Part print with two shaded views. Sizes in mm from the minimum x, y, z corner. Round coordinates to 2 decimals unless told otherwise and drop trailing zeros. Loops run counter-clockwise (first coordinate to the right, second up) from the corner with the lowest first, then second, coordinate; pieces in that order, holes last. Notation, with made-up numbers: M 68.25,13 L 97.25,13 A9 ccw 97.25,26 Z; hole C 56.25,70 d9. An arc over 180 degrees is marked long. Use a Markdown table: item, result. Add a question column.
Item 1: Pin check, flat tips, straight feed: P1, Ø5, axis at x = 185.5, z = 11, coming from the -Y side; P2, Ø10, axis at y = 18.5, z = 2.5, coming from the -X side; P3, Ø5.5, axis at y = 42, z = 2, coming from the +X side. Stop position of each tip, or through.
Item 2: Saw through at C-C on y = 43. Write the cut outline in (x, z), then the cut area to 3 significant figures.
Item 3: Saw through at A-A on x = 175. Write the cut outline in (y, z).
Item 4: Saw through at D-D on x = 67. Write the cut outline in (y, z), then the cut area to 3 significant figures.
Item 5: Wall check: L1, parallel to Y at x = 182.3, z = 3.65; L2, parallel to Z at x = 178.5, y = 80; L3, parallel to X at y = 47.5, z = 4. Give the ranges that are in metal, low to high. Write a range as from..to.
Item 6: Saw through at B-B on z = 11. Write the cut outline in (x, y).
Item 7: Two-plate mould, pull along Y, no slides. Class the marked faces 1 and 2: +Y half, -Y half, draft (parallel to the pull), parting line (faces both ways), or undercut.
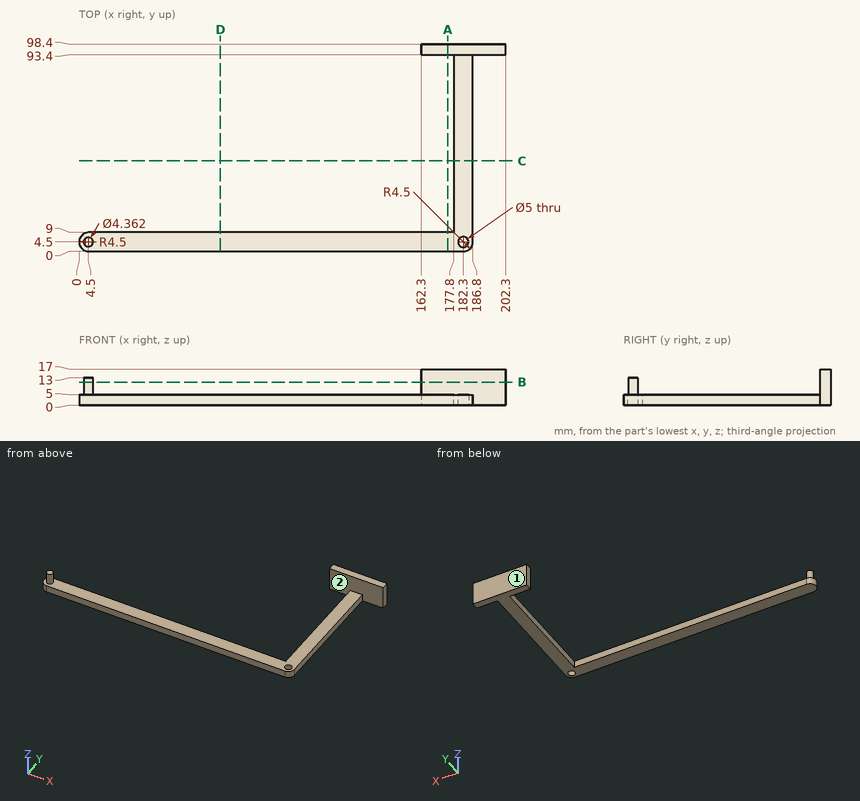
Entries:
| question | item | result |
|---|---|---|
| 1 | P1 | y = 93.4 |
| 1 | P2 | x = 177.8 |
| 1 | P3 | x = 186.8 |
| 2 | outline | M 177.8,0 L 186.8,0 L 186.8,5 L 177.8,5 Z |
| 2 | area | 45.0 mm2 |
| 3 | outline | M 0,0 L 9,0 L 9,5 L 0,5 Z; M 93.4,0 L 98.4,0 L 98.4,17 L 93.4,17 Z |
| 4 | outline | M 0,0 L 9,0 L 9,5 L 0,5 Z |
| 4 | area | 45.0 mm2 |
| 5 | L1 | 0..2, 7..98.4 |
| 5 | L2 | 0..5 |
| 5 | L3 | 177.8..186.8 |
| 6 | outline | C 4.5,4.5 d4.36; M 162.3,93.4 L 202.3,93.4 L 202.3,98.4 L 162.3,98.4 Z |
| 7 | face 1 | +Y half |
| 7 | face 2 | undercut |
